```python
from build123d import *

# Parameters (mm, degrees)
BOSS_EXTRUDE1_DEPTH = 1.5
CHAMFER1_SIZE       = 1.5


with BuildPart() as part:
    # Sketch1 → Boss-Extrude1 (new, symmetric)
    with BuildSketch(Plane.XY):
        Polygon((0, 0), (0, 234), (184, 49), (218, -80), align=None)
    extrude(amount=BOSS_EXTRUDE1_DEPTH, both=True)

    # Chamfer1
    # the kernel refuses this chamfer: 1.5 mm, written as the material it takes off along each edge
    with BuildSketch(Plane(origin=(-2.720279639, 236.735063768, -1.5), x_dir=(0.01949513897586929, 0.01938975984627006, 0.9996219169112969), z_dir=(0.7051879131144355, -0.7090204561204898, 0)), Plane(origin=(-2.720279639, 236.735063768, 1.5), x_dir=(-0.708752387476486, -0.704921293490129, 0.027495876610586337), z_dir=(0.7051879131144355, -0.7090204561204898, 0))) as chamfer1_piece_1:
        Polygon((CHAMFER1_SIZE * 0.999621916911, CHAMFER1_SIZE * 0.0274958766106), (-CHAMFER1_SIZE * 0.0274958766106, CHAMFER1_SIZE * 0.999621916911), (0, 0), align=None)
    extrude(amount=268.638409359, mode=Mode.SUBTRACT)
    with BuildSketch(Plane(origin=(221.621380299, -81.328946899, -1.5), x_dir=(0.3443774504996801, 0.9384285526116285, -0.0274958766105866), z_dir=(-0.9387834907734437, 0.34450770303612605, 0))) as chamfer1_piece_2:
        Polygon((CHAMFER1_SIZE * 0.999621916911, -CHAMFER1_SIZE * 0.0274958766106), (-CHAMFER1_SIZE * 0.0274958766106, -CHAMFER1_SIZE * 0.999621916911), (0, 0), align=None)
    extrude(amount=239.930466195, mode=Mode.SUBTRACT)
    with BuildSketch(Plane(origin=(221.621380299, -81.328946899, 1.5), x_dir=(0.3443774504996801, 0.9384285526116285, 0.0274958766105866), z_dir=(-0.9387834907734437, 0.34450770303612605, 0))) as chamfer1_piece_3:
        Polygon((CHAMFER1_SIZE * 0.999621916911, CHAMFER1_SIZE * 0.0274958766106), (-CHAMFER1_SIZE * 0.0274958766106, CHAMFER1_SIZE * 0.999621916911), (0, 0), align=None)
    extrude(amount=239.930466195, mode=Mode.SUBTRACT)


solid = part.part
```
The listing builds one solid part. Answer for the finished solid, in the listing's coordinates (mm). Give positions to 0.01 mm unless a question says otherwise; leave off trailing zeros. Write each loop counter-clockwise with the first axis right and the second up, starting at its lowest first coordinate (ties: lowest second). Pieces come first, ordered by that corner, then holes. Notation, with made-up numbers: M -1.5,44 L 7.5,44 A25 cw 7.5,59 Z; hole C 50,56.5 d2. An arc over 180 degrees is marked long. Write each question's results on one line, items separated by ' | '.
Q1. Section B-B, the plane y = -25.5 is taken. Write down the section's boundary in (x, z).
Output values:
outline: M 69.49,0 L 73.84,-1.5 L 203.64,-1.5 L 203.64,1.5 L 73.84,1.5 Z
Q2. Consider L1, parallel to Y at x = 180, z = 0.4; L2, parallel to Y at x = 148.5, z = 0.6; L3, parallel to X at y = 92.5, z = -0.25. Determine where each line is inside the solid, lowest interval first. Write a range as from..to.
Output values:
L1: -65.63..52.45 | L2: -53.86..83.84 | L3: 0..140.38
Q3. For a pull along Y with two mould halves and no side action, classify faces 1 (the flat face through (91.073, 141.353, 0.761)), 2 (the flat face through (86, 45, -1.5)), 3 (the flat face through (110.53, -39.75, -0.76)) as released by +Y, released by -Y, zero draft, split by the parting line, or undercut.
Output values:
face 1: released by +Y | face 2: zero draft | face 3: released by -Y
Q4. Section A-A, the plane x = 112 is taken. Write down the section's boundary in (y, z), then the cut area to 3 significant figures.
Output values:
outline: M -41.1,0 L -39.5,-1.5 L 119.26,-1.5 L 121.39,0 L 119.26,1.5 L -39.5,1.5 Z | area: 482 mm2
Q5. Section C-C, the plane y = 93 is taken. Write down the section's boundary in (x, z), then the cut area to 3 significant figures.
Output values:
outline: M 0,-1.5 L 138.12,-1.5 L 140.24,0 L 138.12,1.5 L 0,1.5 Z | area: 418 mm2
Q6. Section D-D, the plane z = -0.85 is taken. Write down the section's boundary in (x, y).
Output values:
outline: M 0,0.91 L 217.74,-79 L 184.43,47.36 L 0,232.79 Z
